Geometry check sheet. Reference: drawing and pictorial views, mm from the part's lowest x, y, z. A direction names the side the tool comes from. Give positions to 0.01 mm unless a question says otherwise; leave off trailing zeros. Write each loop counter-clockwise with the first axis right and the second up, starting at its lowest first coordinate (ties: lowest second). Pieces come first, ordered by that corner, then holes. Notation, with made-up numbers: M 9,35.25 L 21,35.25 A13 cw 21,41.25 Z; hole C 57.25,41.25 d6. An arc over 180 degrees is marked long. Write item = value, one per line. Start each with the question number.
1) Access from +Z, -Z, +X, -X, +Y, -Y to the whole of each face (thin tool, end or side, straight path). Record for the marked faces 1 and 2.
2) Go/stop test with flat-tipped pins: pin 1 (8 mm diameter, centred on y = 9.5, z = 22.5, fed in from -X); pin 2 (3 mm diameter, centred on x = 93, z = 8, fed in from -Y); pin 3 (24 mm diameter, centred on x = 39, z = 20, fed in from +Y). Record where each tip stops, or that it passes through.
3) Cross-section at A-A, the plane z = 8. Record the cut outline in (x, y) (3 decimals).
4) Cross-section at D-D, the plane z = 34.5. Record the cut outline in (x, y).
5) Cross-section at C-C, the plane x = 7. Record the cut outline in (y, z) (3 decimals).
6) Cross-section at B-B, the plane y = 42. Record the cut outline in (x, z).
7) Scan lines: line 1 along X through (y, z) = (1.25, 66) (3 decimals); line 2 along Z through (x, y) = (93, 0.85) (3 decimals); line 3 along Z through (x, y) = (105, 42). Record each from-to range of solid material in increasing order. Write a range as [from, to].
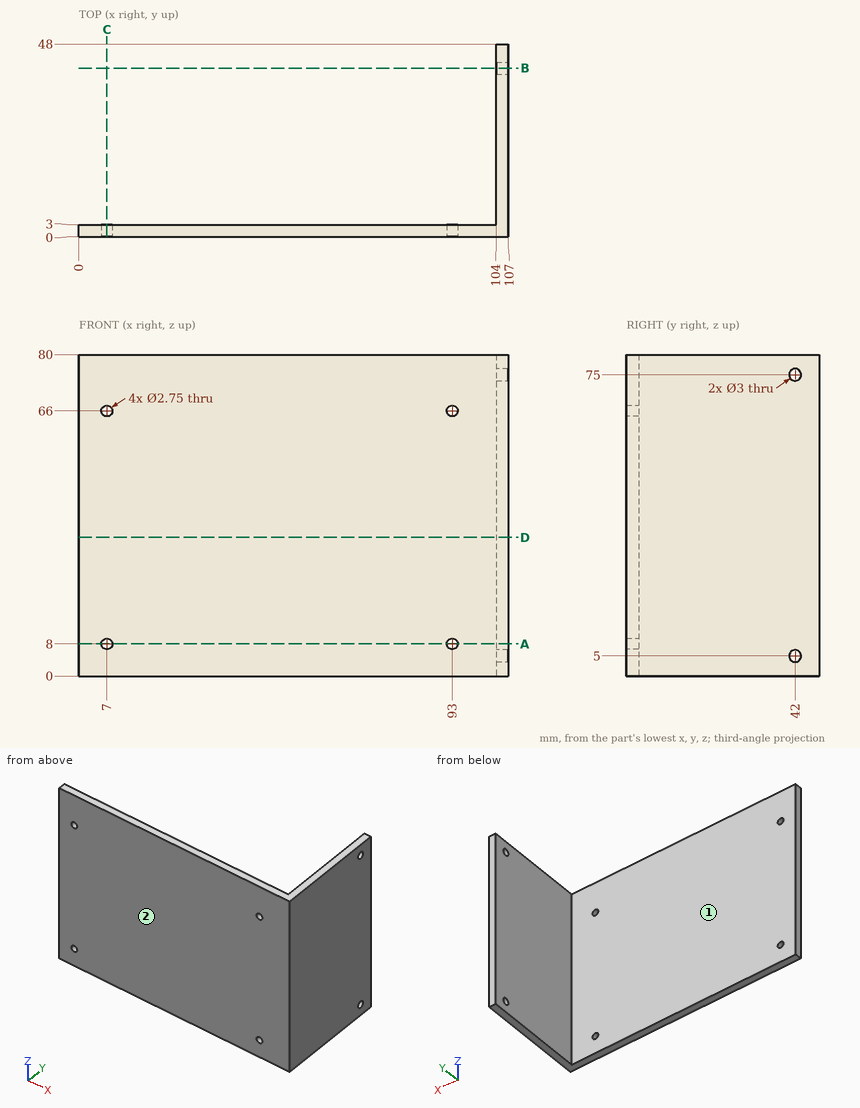
Reply:
q1.face_1 = +Z, -Z, -X, +Y
q1.face_2 = +Z, -Z, +X, -X, -Y
q2.pin_1 = 104
q2.pin_2 = 0
q2.pin_3 = 3
q3.outline = M 0,0 L 5.625,0 L 5.625,3 L 0,3 Z; M 8.375,0 L 91.625,0 L 91.625,3 L 8.375,3 Z; M 94.375,0 L 107,0 L 107,48 L 104,48 L 104,3 L 94.375,3 Z
q4.outline = M 0,0 L 107,0 L 107,48 L 104,48 L 104,3 L 0,3 Z
q5.outline = M 0,0 L 3,0 L 3,6.625 L 0,6.625 Z; M 0,9.375 L 3,9.375 L 3,64.625 L 0,64.625 Z; M 0,67.375 L 3,67.375 L 3,80 L 0,80 Z
q6.outline = M 104,0 L 107,0 L 107,3.5 L 104,3.5 Z; M 104,6.5 L 107,6.5 L 107,73.5 L 104,73.5 Z; M 104,76.5 L 107,76.5 L 107,80 L 104,80 Z
q7.line_1 = [0, 5.625], [8.375, 91.625], [94.375, 107]
q7.line_2 = [0, 6.625], [9.375, 64.625], [67.375, 80]
q7.line_3 = [0, 3.5], [6.5, 73.5], [76.5, 80]
